Read the model definition and answer for the solid it produces. Units are mm, in the model's axes. Coordinates: 2 decimals unless noted, no trailing zeros. Write each loop counter-clockwise with the first axis right and the second up, starting at its lowest first coordinate (ties: lowest second). Pieces come first, ordered by that corner, then holes.
1) The part is cut by section A-A (x = 0). Determine the outline of the cut face in (y, z).
2) Each of these flat-tipped pins is pushed along its axis until it touches: pin 1 Ø2 at (y, z) = (-2, 12.5) entering from -X; pin 2 Ø3 at (x, y) = (6.5, -8) entering from -Z; pin 3 Ø4 at (x, z) = (-3.5, 11) entering from +Y; pin 4 Ø12 at (x, z) = (7.5, 8.5) entering from -Y. Where does it stop, or does it pass through?
3) Find the intervals of material crossed by line 1 (Y direction, x = 0, z = 22); line 2 (Y direction, x = -1.5, z = 15); line 3 (X direction, y = -4.5, z = 19), in increasing order.
4) Determine the mould class of faces 1 (the face through (-1.604, -7.224, 24.158)), 2 (the face through (2.13, 7.3, 0)), 3 (the face through (-2.17, -9.76, 24.16)) for opening direction Y: +Y half, -Y half, draft (parallel to the pull), parting line (faces both ways), or undercut.
5) The part is cut by section C-C (z = 24.5). Determine the outline of the cut face in (x, y), then the cut area to 3 significant figures.
from build123d import *

# Parameters (mm, degrees)
SCHIZZO1_R                   = 10
SCHIZZO1_R_2                 = 7.4
ESTRUSIONE_ESTRUSIONE1_DEPTH = 49
RACCORDO1_R                  = 0.2
RACCORDO2_R                  = 0.05


with BuildPart() as part:
    # Schizzo1 → Estrusione-Estrusione1 (new body)
    with BuildSketch(Plane.XY):
        Circle(SCHIZZO1_R)
        Circle(SCHIZZO1_R_2, mode=Mode.SUBTRACT)
    extrude(amount=ESTRUSIONE_ESTRUSIONE1_DEPTH)

    # Raccordo1
    raccordo1_edges = [part.edges().sort_by_distance(p)[0] for p in [
        (-10, 0, 0),
        (-10, 0, 49),
    ]]
    fillet(raccordo1_edges, radius=RACCORDO1_R)

    # Raccordo2
    raccordo2_edges = [part.edges().sort_by_distance(p)[0] for p in [
        (-7.4, 0, 0),
        (-7.4, 0, 49),
    ]]
    fillet(raccordo2_edges, radius=RACCORDO2_R)


solid = part.part
Reported:
1. outline: (-10, 0.2) arc R0.2 ccw to (-9.8, 0) - (-7.45, 0) arc R0.05 ccw to (-7.4, 0.05) - (-7.4, 48.95) arc R0.05 ccw to (-7.45, 49) - (-9.8, 49) arc R0.2 ccw to (-10, 48.8) - close; (7.4, 0.05) arc R0.05 ccw to (7.45, 0) - (9.8, 0) arc R0.2 ccw to (10, 0.2) - (10, 48.8) arc R0.2 ccw to (9.8, 49) - (7.45, 49) arc R0.05 ccw to (7.4, 48.95) - close
2. pin 1: stops at x = -9.95
2. pin 2: stops at z = 0
2. pin 3: stops at y = 9.89
2. pin 4: stops at y = -9.89
3. line 1: y = -10 to -7.4, 7.4 to 10
3. line 2: y = -9.89 to -7.25, 7.25 to 9.89
3. line 3: x = -8.93 to -5.87, 5.87 to 8.93
4. face 1: undercut
4. face 2: draft
4. face 3: parting line
5. outline: circle Ø20 at (0, 0); hole circle Ø14.8 at (0, 0)
5. area: 142 mm2
